CAD build for the part. Positions are in the model's coordinates, mm. Face numbers are marked on the shaded views. A direction names the side the tool comes from. Give positions to 0.01 mm unless a question says otherwise; leave off trailing zeros. Loops run counter-clockwise (first coordinate to the right, second up) from the corner with the lowest first, then second, coordinate; pieces in that order, holes last.
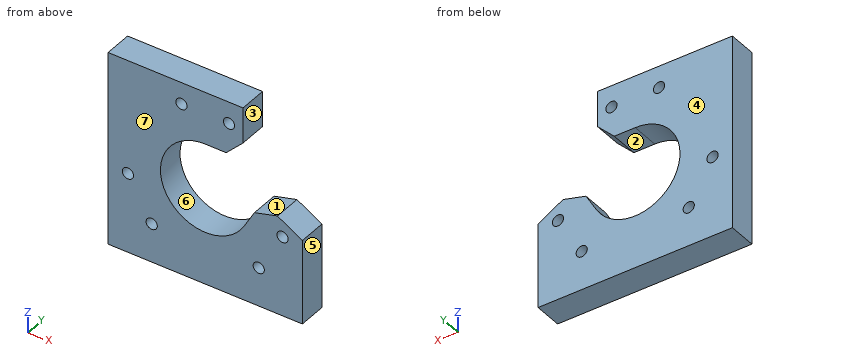
```python
from build123d import *

# Parameters (mm, degrees)
F0_W     = 80
F0_H     = 80
F0_R     = 2
F0_R_2   = 16
F1_DEPTH = 10
F2_W     = 80
F2_H     = 80
F2_W_2   = 69.46222
F2_H_2   = 69.46222
F3_DEPTH = 25
F5_DEPTH = 25


with BuildPart() as f1:
    # F0 (on Front) → F1 (new body)
    with BuildSketch(Plane.XZ):
        Rectangle(F0_W, F0_H)
        with Locations((-19.132686, -20.861216)):
            Circle(F0_R, mode=Mode.SUBTRACT)
        with Locations((-27.632686, -6.138784)):
            Circle(F0_R, mode=Mode.SUBTRACT)
        with Locations((19.132686, -20.861216)):
            Circle(F0_R, mode=Mode.SUBTRACT)
        with Locations((27.632686, -6.138784)):
            Circle(F0_R, mode=Mode.SUBTRACT)
        with Locations((-8.5, 27)):
            Circle(F0_R, mode=Mode.SUBTRACT)
        Circle(F0_R_2, mode=Mode.SUBTRACT)
        with Locations((8.5, 27)):
            Circle(F0_R, mode=Mode.SUBTRACT)
    extrude(amount=F1_DEPTH)

    # F2 (on face) → F3 (cut)
    with BuildSketch(Plane.XZ.offset(10)):
        Rectangle(F2_W, F2_H)
        Rectangle(F2_W_2, F2_H_2, mode=Mode.SUBTRACT)
    extrude(amount=-F3_DEPTH, mode=Mode.SUBTRACT)

    # F4 (on face) → F5 (cut)
    with BuildSketch(Plane.XZ.offset(10)):
        Polygon((17.606406, -1.504809), (25.802559, 0.691343), (41.845802, -8.571228), (36.725588, 37.045255), (13.5, 34.73111), (13.5, 22), (7.5, 16), (0, 16), (13.856406, -8), align=None)
    extrude(amount=-F5_DEPTH, mode=Mode.SUBTRACT)


solid = f1.part
```
1. Saw through at A-A, the plane z = 27. List the corners of the cut face in (x, y).
Responses:
outline: (-34.73, -10) - (-10.5, -10) - (-10.5, 0) - (-34.73, 0) - close; (-6.5, -10) - (6.5, -10) - (6.5, 0) - (-6.5, 0) - close; (10.5, -10) - (13.5, -10) - (13.5, 0) - (10.5, 0) - close
2. Saw through at D-D, the plane y = -5.5. List the corners of the cut face in (x, z).
Responses:
outline: (-34.73, -34.73) - (34.73, -34.73) - (34.73, -4.46) - (25.8, 0.69) - (17.61, -1.5) - (13.86, -8) arc R16 cw (long way) to (0, 16) - (7.5, 16) - (13.5, 22) - (13.5, 34.73) - (-34.73, 34.73) - close; hole circle Ø4 at (-27.63, -6.14); hole circle Ø4 at (-19.13, -20.86); hole circle Ø4 at (-8.5, 27); hole circle Ø4 at (8.5, 27); hole circle Ø4 at (19.13, -20.86); hole circle Ø4 at (27.63, -6.14)
3. Saw through at B-B, the plane x = 8.5. List the corners of the cut face in (y, z).
Responses:
outline: (-10, -34.73) - (0, -34.73) - (0, -13.56) - (-10, -13.56) - close; (-10, 17) - (0, 17) - (0, 25) - (-10, 25) - close; (-10, 29) - (0, 29) - (0, 34.73) - (-10, 34.73) - close
4. Tool access for the marked faces 1, 2, 3 and 4: list every direction of +Z, -Z, +X, -X, +Y, -Y with a clear straight run to the whole face (end or side of a thin tool).
Responses:
face 1: +Z, +Y, -Y
face 2: +X, +Y, -Y
face 3: +Z, +X, +Y, -Y
face 4: +Z, -Z, +X, -X, +Y
5. Probe line 1 along X through (y, z) = (-8.75, -19.5); line 2 along X through (y, z) = (-7.5, 26.5); line 3 along Z through (x, y) = (-8.5, -5.5). List the from-to ranges inside material, lowest first.
Responses:
line 1: x = -34.73 to -20.6, -17.67 to 17.67, 20.6 to 34.73
line 2: x = -34.73 to -10.44, -6.56 to 6.56, 10.44 to 13.5
line 3: z = -34.73 to -13.56, 13.56 to 25, 29 to 34.73
6. Pull direction X, two halves, no side cores. Call the marked faces 5, 6 and 7: released by +X, released by -X, zero draft, split by the parting line, or undercut.
Responses:
face 5: released by +X
face 6: undercut
face 7: zero draft
7. Saw through at C-C, the plane x = -12.5. List the corners of the cut face in (y, z), and give its area (3 significant figures).
Responses:
outline: (-10, -34.73) - (0, -34.73) - (0, -9.99) - (-10, -9.99) - close; (-10, 9.99) - (0, 9.99) - (0, 34.73) - (-10, 34.73) - close
area: 495 mm2
8. Drop flat-ended pins along their axis: pin 1 (12 mm diameter, centred on x = -5.5, z = 6.5, fed in from -Y); pin 2 (4 mm diameter, centred on y = -6, z = 17, fed in from +X). Give the stop position or say it passes through.
Responses:
pin 1: passes through
pin 2: stops at x = 10.5
